Here's how the part is built. I have some questions about the finished solid (model axes, mm). Face numbers are marked on the shaded views. A direction names the side the tool comes from. Coordinates: 2 decimals unless noted, no trailing zeros. Write each loop counter-clockwise with the first axis right and the second up, starting at its lowest first coordinate (ties: lowest second). Pieces come first, ordered by that corner, then holes.
Item 1: If we section it at A-A (x = -46): Please give me the cut outline in (y, z).
Item 2: I'm going to push flat-ended pins straight in: pin 1 Ø5.5 at (x, z) = (-46, -174.4) entering from -Y; pin 2 Ø5.5 at (x, y) = (-46.5, 48.5) entering from -Z; pin 3 Ø1.8 at (x, y) = (-1, 37.5) entering from -Z; pin 4 Ø0.7 at (y, z) = (46, -134.5) entering from -X. Where does each tip first touch, or does it pass through?
Item 3: If we section it at B-B (z = -108): Please give me the cut outline in (x, y).
Item 4: For the marked faces 1 and 2, which set-ups out of +Z, -Z, +X, -X, +Y, -Y let a thin tool reach every point of the face, with its end or its side?
Item 5: If I drill on line 1 (X direction, y = 24, z = -142); line 2 (X direction, y = 46, z = -134); line 3 (Z direction, x = -46, y = 22), over which ranges is the centre line in solid material (lowest first)?
Item 6: If we section it at D-D (z = -155.5): Please give me the cut outline in (x, y).
Item 7: If we section it at C-C (y = 45.5): Please give me the cut outline in (x, z).
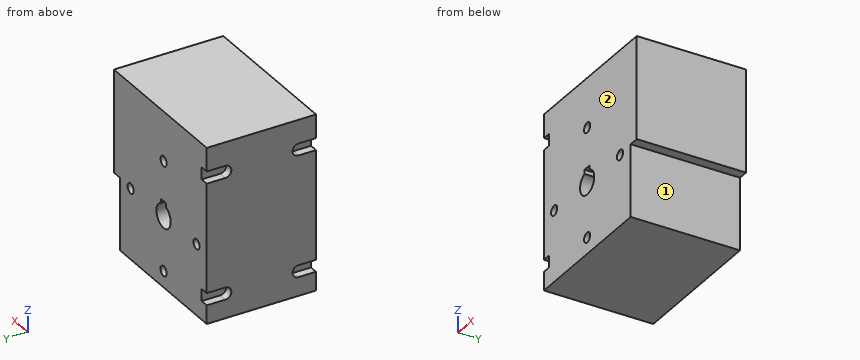
from build123d import *

# Parameters (mm, degrees)
PAD002_DEPTH           = 65
SKETCH004_R            = 3
HOLE001_DEPTH          = 72
POCKET_DEPTH           = 72
POCKET001_DEPTH        = 5
LINEARPATTERN_COUNT    = 2
LINEARPATTERN_PITCH    = 72
POCKET002_DEPTH        = 5
LINEARPATTERN001_COUNT = 2
LINEARPATTERN001_PITCH = 72


with BuildPart() as part:
    # Sketch003 → Pad002 (new body)
    with BuildSketch(Plane.XZ):
        Polygon((3, -80), (-88.623817, -80), (-88.563461, -184.210968), (-3, -184), (-3, -141), (3, -141), align=None)
    extrude(amount=PAD002_DEPTH)

    # Sketch004 (on Face8 of Pad002) → Hole001 (cut)
    with BuildSketch(Plane.XZ.offset(65)):
        with Locations((-46, -109.40177)):
            Circle(SKETCH004_R)
        with Locations((-13.507946, -142)):
            Circle(SKETCH004_R)
        with Locations((-45.999997, -174.401768)):
            Circle(SKETCH004_R)
        with Locations((-78.507649, -142)):
            Circle(SKETCH004_R)
    extrude(amount=-HOLE001_DEPTH, mode=Mode.SUBTRACT)

    # Sketch005 (on Face5 of Hole001) → Pocket (cut)
    with BuildSketch(Plane.XZ.offset(65)):
        with BuildLine():
            ThreePointArc((-48.547432, -135.480744), (-45.913728, -148.984728), (-43.457714, -135.447299))
            Line((-43.457714, -132.991287), (-43.457714, -135.447299))
            Line((-48.547432, -132.991287), (-43.457714, -132.991287))
            Line((-48.547432, -135.480744), (-48.547432, -132.991287))
        make_face()
    extrude(amount=-POCKET_DEPTH, mode=Mode.SUBTRACT)

    # Sketch007 (on Face3 of Pocket) → Pocket001 (cut)
    with BuildSketch(Plane(origin=(-88.670121, 0, -0.051355), x_dir=(0.000579, 0, -1), z_dir=(-1, 0, -0.000579))):
        with BuildLine():
            Line((94, 65.961746), (101.060434, 65.961746))
            Line((101.060434, 65.961746), (101.060434, 54.602297))
            ThreePointArc((94, 54.553143), (97.554966, 51.02284), (101.060434, 54.602297))
            Line((94, 54.553143), (94, 65.961746))
        make_face()
    pocket001 = extrude(amount=-POCKET001_DEPTH, mode=Mode.SUBTRACT)

    # LinearPattern: Pocket001 ×2
    with Locations(*[Vector(0.000579, 0, -1) * (i * LINEARPATTERN_PITCH) for i in range(1, LINEARPATTERN_COUNT)]):
        add(pocket001, mode=Mode.SUBTRACT)

    # Sketch008 (on Face3 of LinearPattern) → Pocket002 (cut)
    with BuildSketch(Plane(origin=(-88.670121, 0, -0.051355), x_dir=(0.000579, 0, -1), z_dir=(-1, 0, -0.000579))):
        with BuildLine():
            ThreePointArc((101.128495, 11.00325), (97.494061, 14.625529), (93.920682, 10.943006))
            Line((93.920682, -1.640862), (93.920682, 10.943006))
            Line((101.128495, -1.640862), (93.920682, -1.640862))
            Line((101.128495, 11.00325), (101.128495, -1.640862))
        make_face()
    pocket002 = extrude(amount=-POCKET002_DEPTH, mode=Mode.SUBTRACT)

    # LinearPattern001: Pocket002 ×2
    with Locations(*[Vector(0.000579, 0, -1) * (i * LINEARPATTERN001_PITCH) for i in range(1, LINEARPATTERN001_COUNT)]):
        add(pocket002, mode=Mode.SUBTRACT)


with BuildPart() as part_1:
    # Body002 placement: moved
    add(part.part.moved(Location((0, 66, 0))))


solid = part_1.part
Answer list:
1. outline: (1, -184.11) - (66, -184.11) - (66, -177.4) - (1, -177.4) - close; (1, -171.4) - (66, -171.4) - (66, -148.98) - (1, -148.98) - close; (1, -132.99) - (66, -132.99) - (66, -112.4) - (1, -112.4) - close; (1, -106.4) - (66, -106.4) - (66, -80) - (1, -80) - close
2. pin 1: passes through
2. pin 2: stops at z = -184.11
2. pin 3: stops at z = -141
2. pin 4: stops at x = -88.59
3. outline: (-88.61, 1) - (-48.65, 1) - (-48.65, 66) - (-88.61, 66) - close; (-43.35, 1) - (3, 1) - (3, 66) - (-43.35, 66) - close
4. face 1: -Z, +X, +Y, -Y
4. face 2: +Z, -Z, +X, -X, -Y
5. line 1: x = -88.59 to -81.51, -75.51 to -52.96, -38.96 to -16.51, -10.51 to -3
5. line 2: x = -88.59 to -48.55, -43.46 to 3
5. line 3: z = -184.11 to -177.4, -171.4 to -148.98, -132.99 to -112.4, -106.4 to -80
6. outline: (-88.58, 1) - (-3, 1) - (-3, 66) - (-88.58, 66) - close
7. outline: (-88.62, -80) - (-88.56, -184.21) - (-3, -184) - (-3, -141) - (3, -141) - (3, -80) - close; hole circle Ø6 at (-78.51, -142); hole circle Ø6 at (-46, -174.4); hole circle Ø6 at (-46, -109.4); hole (-48.55, -135.48) arc R7 ccw (long way) to (-43.46, -135.45) - (-43.46, -132.99) - (-48.55, -132.99) - close; hole circle Ø6 at (-13.51, -142)
